Answer from the drawing. Dimensions are ordinates in mm from the lowest x, y and z of the part. Round coordinates to 2 decimals unless told otherwise and drop trailing zeros. Loops run counter-clockwise (first coordinate to the right, second up) from the corner with the lowest first, then second, coordinate; pieces in that order, holes last. Notation, with made-up numbers: (-5.5, -21.5) -> (12.5, -21.5) arc R33 ccw to (12.5, 13.5) -> close; hole circle Ø6 at (-37, 42.5). An arc over 180 degrees is marked (long way). One line per question, with ' | ' between items.
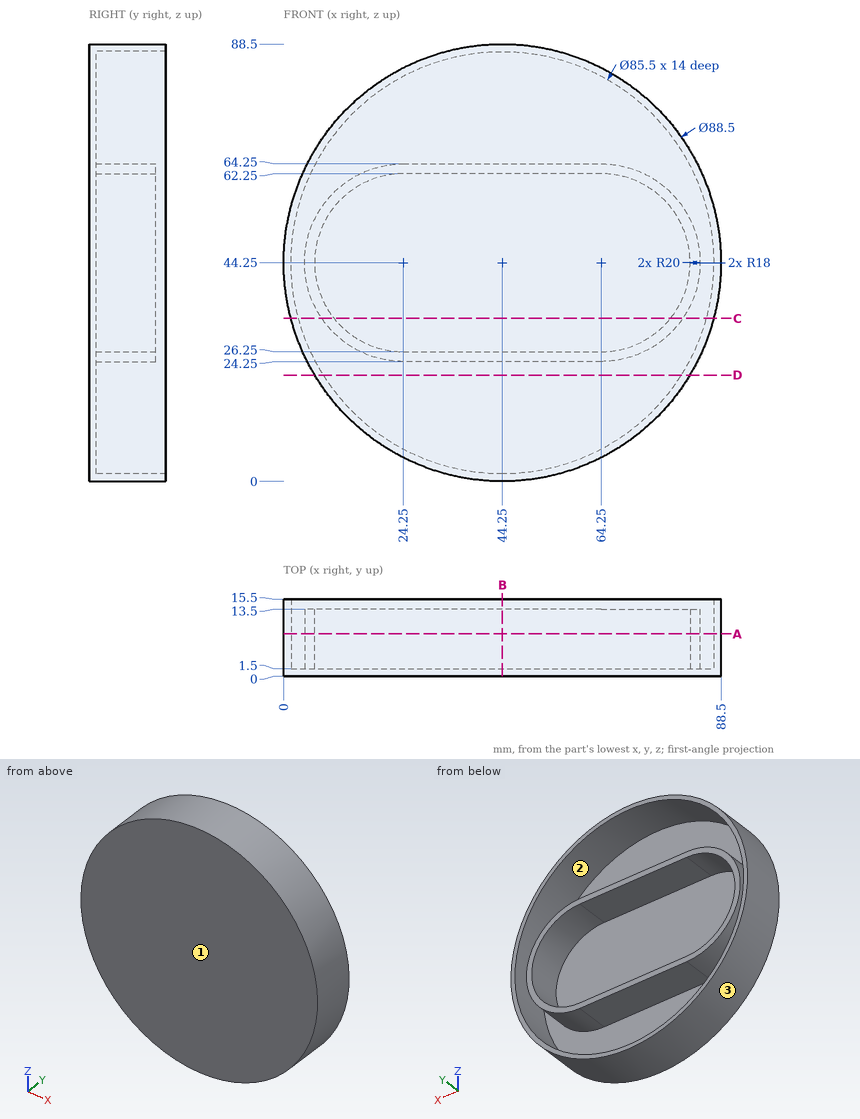
Q1. A cutting plane is placed at C-C on z = 33. Give the vertices of the cut face in (x, y).
Numbers:
outline: (1.45, 0) -> (87.05, 0) -> (87.05, 15.5) -> (85.49, 15.5) -> (85.49, 1.5) -> (80.79, 1.5) -> (80.79, 13.5) -> (78.3, 13.5) -> (78.3, 1.5) -> (10.2, 1.5) -> (10.2, 13.5) -> (7.71, 13.5) -> (7.71, 1.5) -> (3.01, 1.5) -> (3.01, 15.5) -> (1.45, 15.5) -> close
Q2. Find the intervals of material crossed by line 1 (X direction, y = 11.5, z = 44.25); line 2 (Z direction, x = 6, y = 13.25); line 3 (Z direction, x = 10.5, y = 5), in increasing order. Write a range as from..to.
Numbers:
line 1: 0..1.5, 4.25..6.25, 82.25..84.25, 87..88.5 | line 2: 22..25.16, 36.07..52.43, 63.34..66.5 | line 3: 15.63..18.01, 29.73..32.63, 55.87..58.77, 70.49..72.87
Q3. A cutting plane is placed at A-A on y = 8.5. Give the vertices of the cut face in (x, z).
Numbers:
outline: circle Ø88.5 at (44.25, 44.25); (24.25, 24.25) -> (64.25, 24.25) arc R20 ccw to (64.25, 64.25) -> (24.25, 64.25) arc R20 ccw to start; hole circle Ø85.5 at (44.25, 44.25); hole (24.25, 26.25) -> (64.25, 26.25) arc R18 ccw to (64.25, 62.25) -> (24.25, 62.25) arc R18 ccw to start
Q4. A cutting plane is placed at D-D on z = 21.5. Give the vertices of the cut face in (x, y), plus the area to 3 significant figures.
Numbers:
outline: (6.3, 0) -> (82.2, 0) -> (82.2, 15.5) -> (80.44, 15.5) -> (80.44, 1.5) -> (8.06, 1.5) -> (8.06, 15.5) -> (6.3, 15.5) -> close | area: 163 mm^2
Q5. For a pull along X with two mould halves and no side action, classify the marked faces 1, 2 and 3 as pulls with the +X half, pulls with the -X half, needs draft (parallel to the pull), parting line crosses it, or undercut.
Numbers:
face 1: needs draft | face 2: undercut | face 3: parting line crosses it
Q6. A cutting plane is placed at B-B on x = 44.25. Give the vertices of the cut face in (y, z).
Numbers:
outline: (0, 0) -> (15.5, 0) -> (15.5, 1.5) -> (1.5, 1.5) -> (1.5, 24.25) -> (13.5, 24.25) -> (13.5, 26.25) -> (1.5, 26.25) -> (1.5, 62.25) -> (13.5, 62.25) -> (13.5, 64.25) -> (1.5, 64.25) -> (1.5, 87) -> (15.5, 87) -> (15.5, 88.5) -> (0, 88.5) -> close
Q7. Given pin 1 Ø6 at (x, y) = (17, 8) entering from +Z; pin 2 Ø8 at (y, z) = (3, 40) entering from -X; pin 3 Ø2 at (y, z) = (10, 39.5) entering from +X; pin 4 Ø1 at (x, z) = (10, 14) entering from +Y, each flat-ended and moving along its own axis, determine where each tip first touches the part or whether it passes through.
Numbers:
pin 1: z = 81.26 | pin 2: x = 0 | pin 3: x = 88.34 | pin 4: through
